from build123d import *

# Parameters (mm, degrees)
BOSS_EXTRUDE1_DEPTH = 4
BOSS_EXTRUDE2_DEPTH = 29
CHAMFER1_SIZE       = 4
CHAMFER2_SIZE       = 6
CUT_EXTRUDE1_REACH  = 48.626
SKETCH3_R           = 2.5
CUT_EXTRUDE2_REACH  = 48.626
SKETCH4_R           = 2.5
SKETCH5_W           = 5
SKETCH5_H           = 3
BOSS_EXTRUDE3_DEPTH = 27
FILLET1_R           = 2


with BuildPart() as part:
    # Sketch1 → Boss-Extrude1 (new, symmetric)
    with BuildSketch(Plane.XY):
        Polygon((0, 0), (0, 35), (8, 35), (8, 8), (30, 8), (30, 0), align=None)
    extrude(amount=BOSS_EXTRUDE1_DEPTH, both=True)

    # Sketch2 → Boss-Extrude2 (add)
    with BuildSketch(Plane(origin=(30, 0, 0), x_dir=(0, 0, -1), z_dir=(1, 0, 0))):
        Polygon((-4, 6.5), (-7, 6.5), (-7, 1.5), (-4, 0), align=None)
        Polygon((4, 0), (4, 6.5), (7, 6.5), (7, 1.5), align=None)
    extrude(amount=-BOSS_EXTRUDE2_DEPTH)

    # Chamfer1
    # the kernel refuses this chamfer: 4 mm, written as the material it takes off along each edge
    with BuildSketch(Plane(origin=(30, 16.786731952, -7), x_dir=(0.027495876610586487, 0, 0.9996219169112968), z_dir=(0, -1, 0))) as chamfer1_piece_1:
        Polygon((CHAMFER1_SIZE * 0.999621916911, CHAMFER1_SIZE * 0.0274958766106), (-CHAMFER1_SIZE * 0.0274958766106, CHAMFER1_SIZE * 0.999621916911), (0, 0), align=None)
    extrude(amount=25.573463904, mode=Mode.SUBTRACT)
    with BuildSketch(Plane(origin=(1, 16.786731952, -7), x_dir=(-0.02749587661058638, 0, 0.9996219169112968), z_dir=(0, -1, 0))) as chamfer1_piece_2_section:
        Polygon((CHAMFER1_SIZE * 0.999621916911, -CHAMFER1_SIZE * 0.0274958766106), (-CHAMFER1_SIZE * 0.0274958766106, -CHAMFER1_SIZE * 0.999621916911), (0, 0), align=None)
    chamfer1_piece_2 = extrude(amount=25.573463904, mode=Mode.PRIVATE)
    chamfer1_piece_2 = split(chamfer1_piece_2, bisect_by=Plane(origin=(2.407836441, 4, -4), z_dir=(0, 0, -1)), keep=Keep.TOP, mode=Mode.PRIVATE)
    add(chamfer1_piece_2, mode=Mode.SUBTRACT)
    with BuildSketch(Plane(origin=(30, 16.786731952, 7), x_dir=(0.027495876610586487, 0, -0.9996219169112968), z_dir=(0, -1, 0))) as chamfer1_piece_3:
        Polygon((CHAMFER1_SIZE * 0.999621916911, -CHAMFER1_SIZE * 0.0274958766106), (-CHAMFER1_SIZE * 0.0274958766106, -CHAMFER1_SIZE * 0.999621916911), (0, 0), align=None)
    extrude(amount=25.573463904, mode=Mode.SUBTRACT)
    with BuildSketch(Plane(origin=(1, 16.786731952, 7), x_dir=(-0.02749587661058638, 0, -0.9996219169112968), z_dir=(0, -1, 0))) as chamfer1_piece_4_section:
        Polygon((CHAMFER1_SIZE * 0.999621916911, CHAMFER1_SIZE * 0.0274958766106), (-CHAMFER1_SIZE * 0.0274958766106, CHAMFER1_SIZE * 0.999621916911), (0, 0), align=None)
    chamfer1_piece_4 = extrude(amount=25.573463904, mode=Mode.PRIVATE)
    chamfer1_piece_4 = split(chamfer1_piece_4, bisect_by=Plane(origin=(2.407836441, 4, 4), z_dir=(0, 0, 1)), keep=Keep.TOP, mode=Mode.PRIVATE)
    add(chamfer1_piece_4, mode=Mode.SUBTRACT)

    # Chamfer2
    chamfer2_edges = [part.edges().sort_by_distance(p)[0] for p in [
        (8, 8, 0),
    ]]
    chamfer(chamfer2_edges, length=CHAMFER2_SIZE)

    # Sketch3 → Cut-Extrude1 (cut, up to next)
    with BuildSketch(Plane.XZ, mode=Mode.PRIVATE) as cut_extrude1_sk1:
        with Locations((22, 0)):
            Circle(SKETCH3_R)
    cut_extrude1_tool1 = extrude(cut_extrude1_sk1.sketch, amount=-CUT_EXTRUDE1_REACH, mode=Mode.PRIVATE) & part.part
    add(cut_extrude1_tool1.solids().sort_by_distance((22, 0, 0))[0], mode=Mode.SUBTRACT)

    # Sketch4 → Cut-Extrude2 (cut, up to next)
    with BuildSketch(Plane.ZY, mode=Mode.PRIVATE) as cut_extrude2_sk1:
        with Locations((0, 25)):
            Circle(SKETCH4_R)
    cut_extrude2_tool1 = extrude(cut_extrude2_sk1.sketch, amount=-CUT_EXTRUDE2_REACH, mode=Mode.PRIVATE) & part.part
    add(cut_extrude2_tool1.solids().sort_by_distance((0, 25, 0))[0], mode=Mode.SUBTRACT)

    # Sketch5 → Boss-Extrude3 (add)
    with BuildSketch(Plane(origin=(0, 35, 0), x_dir=(1, 0, 0), z_dir=(0, 1, 0))):
        with Locations((4, 5.5)):
            Rectangle(SKETCH5_W, SKETCH5_H)
        with Locations((4, -5.5)):
            Rectangle(SKETCH5_W, SKETCH5_H)
    extrude(amount=-BOSS_EXTRUDE3_DEPTH)

    # Fillet1
    fillet1_edges = [part.edges().sort_by_distance(p)[0] for p in [
        (4, 8, -7),
        (4, 35, -7),
        (4, 8, 7),
        (4, 35, 7),
    ]]
    fillet(fillet1_edges, radius=FILLET1_R)


solid = part.part
Input: part model. Units: mm. Frame: model coordinates. A direction names the side the tool comes from. Round coordinates to 2 decimals unless told otherwise and drop trailing zeros. Loops run counter-clockwise (first coordinate to the right, second up) from the corner with the lowest first, then second, coordinate; pieces in that order, holes last. Notation, with made-up numbers: M 19,-8.5 L 31,-8.5 A14 cw 31,18.5 Z; hole C -35,10.25 d10. An arc over 180 degrees is marked long. Answer as CSV lines item,"result". Start each with the question number.
(1) First-contact query: pin 1 (2.5 mm diameter, centred on x = 22, z = -5, fed in from +Y); pin 2 (3 mm diameter, centred on y = 25, z = 0, fed in from -X); pin 3 (4 mm diameter, centred on y = 22.5, z = 1, fed in from +X); pin 4 (1.5 mm diameter, centred on y = 21, z = -5, fed in from +X). Flat tips, straight axial feed; report the tip coordinate or a pass-through.
(2) Reachability of faces 1 (the flat face through (3, 3, 5)), 2 (the cylindrical face through (4.04, 8.57, 6.4)), 3 (the flat face through (6.5, 22, -5)) from +Z, -Z, +X, -X, +Y, -Y: full face, straight path, thin tool, end or side. Return the list, or none.
(3) Draft query along Z for faces 4 (the cylindrical face through (3.94, 27.48, -0.33)), 5 (the flat face through (4, 22, 7)), 6 (the flat face through (15, 0, 0)). Return one class per face: released by +Z, released by -Z, zero draft, split by the parting line, or undercut.
(4) Section C-C, the plane x = 3.5. Output: boundary loops of the cut face in (y, z).
(5) Section B-B, the plane y = 25. Output: boundary loops of the cut face in (x, z).
(6) Section D-D, the plane x = 22. Output: boundary loops of the cut face in (y, z), plus the area to 3 significant figures.
(7) Section A-A, the plane z = 0. Output: boundary loops of the cut face in (x, y).
(8) Line query: line 1 (Z direction, x = 22, y = 3); line 2 (Y direction, x = 4, z = 0); line 3 (Z direction, x = 3, y = 7.5). Output: solid intervals per line, ascending. Write a range as [from, to].
Values found:
1,pin 1,"stops at y = 8"
1,pin 2,"passes through"
1,pin 3,"stops at x = 8"
1,pin 4,"stops at x = 6.5"
2,face 1,"+Z, -X, -Y"
2,face 2,"+Z, +X, -X"
2,face 3,"-Z, +X, +Y"
3,face 4,"undercut"
3,face 5,"released by +Z"
3,face 6,"zero draft"
4,outline,"M 0,-4 L 0.75,-5.5 L 6.5,-5.5 L 6.5,-4 L 8,-4 L 8,-5 A2 ccw 10,-7 L 33,-7 A2 ccw 35,-5 L 35,5 A2 ccw 33,7 L 10,7 A2 ccw 8,5 L 8,4 L 6.5,4 L 6.5,5.5 L 0.75,5.5 L 0,4 Z; hole C 25,0 d5"
5,outline,"M 0,-4 L 1.5,-4 L 1.5,-7 L 6.5,-7 L 6.5,-4 L 8,-4 L 8,-2.5 L 0,-2.5 Z; M 0,2.5 L 8,2.5 L 8,4 L 6.5,4 L 6.5,7 L 1.5,7 L 1.5,4 L 0,4 Z"
6,outline,"M 0,-4 L 1.5,-7 L 6.5,-7 L 6.5,-4 L 8,-4 L 8,-2.5 L 0,-2.5 Z; M 0,2.5 L 8,2.5 L 8,4 L 6.5,4 L 6.5,7 L 1.5,7 L 0,4 Z"
6,area,"58.5 mm²"
7,outline,"M 0,0 L 19.5,0 L 19.5,8 L 14,8 L 8,14 L 8,22.5 L 0,22.5 Z; M 0,27.5 L 8,27.5 L 8,35 L 0,35 Z; M 24.5,0 L 30,0 L 30,8 L 24.5,8 Z"
8,line 1,"z = [-7, -2.5], [2.5, 7]"
8,line 2,"y = [0, 22.5], [27.5, 35]"
8,line 3,"z = [-4, 4]"
